Source: CAD feature listing. Evaluate the final solid. Frame: model axes, mm. A direction names the side the tool comes from. Round coordinates to 2 decimals unless told otherwise and drop trailing zeros. Loops run counter-clockwise (first coordinate to the right, second up) from the corner with the lowest first, then second, coordinate; pieces in that order, holes last. Notation, with made-up numbers: (84.5, -36) - (140.5, -36) arc R15 cw to (140.5, -14) - close; hole circle Ø5 at (81, 21.5). An arc over 180 degrees is marked (long way). One line per question, with ' | ' between items. Start each with the question number.
1. Pin query (flat end, axial travel): pin 1 (6.5 mm diameter, centred on x = 0, z = -62.5, fed in from +Y); pin 2 (1 mm diameter, centred on x = 4.5, y = -22, fed in from -Z); pin 3 (4 mm diameter, centred on x = -22.5, y = -22.5, fed in from -Z); pin 4 (3 mm diameter, centred on y = 1, z = -37.5, fed in from +X). Return the tip coordinate at first contact, or that it passes through.
2. Cut plane D-D (x = 22.5). Return loops of the section in (y, z), then the cut area to 3 significant figures.
3. Access query for faces 4 (the flat face through (-27.5, -9.6, 0.4)), 5 (the flat face through (-27.5, -29, -61)), 6 (the flat face through (-14, 27.5, -37)). Directions: +Z, -Z, +X, -X, +Y, -Y. A direction counts if a zero-diameter tool reaches every point of the face in a straight line with its end or side. Return the directions, or none.
4. Ray query, line 1 (Z direction, x = 0, y = -28); line 2 (Y direction, x = -21, z = -20.5); line 3 (Z direction, x = -13.5, y = 21.5). Return the intervals inside material, ascending.
5. Cut plane C-C (z = -12.5). Return loops of the section in (x, y), then the cut area to 3 significant figures.
6. Cut plane B-B (y = 0). Return loops of the section in (x, z), then the cut area to 3 significant figures.
7. Mould query, pull axis Z, two halves, no side actions, for faces 1 (the flat face through (-19, 6, 0)), 2 (the cylindrical face through (0, -28, -65)), 3 (the flat face through (-27.5, 0, -37)). Classes: pulls with the +Z half, pulls with the -Z half, needs draft (parallel to the pull), parting line crosses it, or undercut.
8. Cut plane A-A (x = -22.5). Return loops of the section in (y, z).
Autodesk Inventor part; units mm, degrees
ref_plane "YZ Plane" through (0, 0, 0) normal (1, 0, 0) x (0, 1, 0)
ref_plane "XZ Plane" through (0, 0, 0) normal (0, 1, 0) x (-1, 0, 0)
ref_plane "XY Plane" through (0, 0, 0) normal (0, 0, 1) x (1, 0, 0)
sketch "Sketch1" plane through (0, 0, 0) normal (0, 0, 1) x (1, 0, 0)
  line L0 (-27.5, 27.5) -> (27.5, 27.5)
  line L1 (27.5, 27.5) -> (27.5, -27.5)
  line L2 (27.5, -27.5) -> (-27.5, -27.5)
  line L3 (-27.5, -27.5) -> (-27.5, 27.5)
  circle A0 centre (-22.5, 22.5) radius 2.5
  circle A1 centre (22.5, 22.5) radius 2.5
  circle A2 centre (-22.5, -22.5) radius 2.5
  circle A3 centre (22.5, -22.5) radius 2.5
  circle A4 centre (0, 0) radius 19.25
  dimension "d1" = 55
  dimension "d2" = 55
  dimension "d3" = 27.5
  dimension "d4" = 27.5
  dimension "d5" = 38.5
  dimension "d6" = 5
  dimension "d7" = 5
  dimension "d8" = 5
  dimension "d9" = 5
  dimension "d10" = 5
  dimension "d11" = 5
  dimension "d12" = 5
  dimension "d13" = 5
  dimension "d14" = 5
  dimension "d15" = 5
  dimension "d16" = 5
  dimension "d17" = 5
extrude "Extrusion1" add sketch "Sketch1" along normal blind 2
sketch "Sketch2" plane through (27.5, -27.5, 0) normal (1, 0, 0) x (0, 0, -1)
  line L0 (0, 0) -> (-2, 0)
  line L1 (0, 0) -> (75, 0)
  line L2 (75, 0) -> (75, -2)
  line L3 (75, -2) -> (-2, -2)
  line L4 (-2, -2) -> (-2, 0)
  point P0 (0, 27.5)
  dimension "d20" = 75
  dimension "d21" = 2
  dimension "d22" = 77
extrude "Extrusion2" add sketch "Sketch2" against normal blind 55
sketch "Sketch3" plane through (-27.5, -27.5, 0) normal (-1, 0, 0) x (0, 0, 1)
  line L0 (-75, -2) -> (2, -2)
  line L1 (-36.5, -2) -> (-36.5, 55)
  line L2 (0, 0) -> (-75, 0)
  line L3 (-36.5, 55) -> (-46.5, 55)
  line L4 (-46.5, 55) -> (-46.5, -2)
  line L5 (-46.5, -2) -> (-26.5, -2)
  line L6 (-26.5, -2) -> (-26.5, 55)
  line L7 (-26.5, 55) -> (-36.5, 55)
  point P0 (0, 27.5)
  dimension "d25" = 57
  dimension "d26" = 10
  dimension "d27" = 57
  dimension "d28" = 20
  dimension "d29" = 57
extrude "Extrusion3" add sketch "Sketch3" along normal blind 2
sketch "Sketch4" plane through (-27.5, 27.5, -26.5) normal (0, 1, 0) x (1, 0, 0)
  line L0 (-2, 0) -> (-2, 20)
  line L1 (-2, 20) -> (27.5, 20)
  line L2 (27.5, 20) -> (27.5, 0)
  line L3 (0, 0) -> (-2, 0)
  line L4 (27.5, 0) -> (-2, 0)
  line L5 (-2, 0) -> (-2, 20)
  point P0 (27.5, -26.5)
  dimension "d32" = 29.5
  dimension "d33" = 20
extrude "Extrusion4" add sketch "Sketch4" along normal blind 2
sketch "Sketch5" plane through (27.5, -27.5, 0) normal (0, 1, 0) x (1, 0, 0)
  line L0 (0, 75) -> (0, 0)
  line L1 (0, 37.5) -> (-27.5, 37.5)
  line L2 (-27.5, 37.5) -> (-27.5, 62.5)
  line L3 (-27.5, 26.5) -> (-27.5, 46.5)
  line L4 (-27.5, 37.5) -> (-27.5, 12.5)
  circle A0 centre (-27.5, 62.5) radius 2.5
  circle A1 centre (-27.5, 12.5) radius 2.5
  point P0 (-27.5, 0)
  dimension "d36" = 27.5
  dimension "d37" = 25
  dimension "d38" = 25
  dimension "d39" = 5
  dimension "d40" = 5
extrude "Extrusion5" cut sketch "Sketch5" against normal blind 2
equation "\"BendRadius\" = Thickness"
equation "\"BendReliefWidth\" = Thickness"
equation "\"BendReliefDepth\" = 0.5 * Thickness"
equation "\"CornerReliefSize\" = 4 * Thickness"
equation "\"MinimumRemnant\" = 2 * Thickness"
equation "\"TransitionRadius\" = BendRadius"
equation "\"JacobiRadiusSize\" = Thickness"
equation "\"GapSize\" = Thickness"
properties part number "MotorClamp"
Answers follow:
1) pin 1: stops at y = -27.5 | pin 2: stops at z = 0 | pin 3: passes through | pin 4: stops at x = -27.5
2) outline: (-29.5, -75) - (-27.5, -75) - (-27.5, 0) - (-25, 0) - (-25, 2) - (-29.5, 2) - close; (-20, 0) - (20, 0) - (20, 2) - (-20, 2) - close; (25, 0) - (27.5, 0) - (27.5, 2) - (25, 2) - close | area: 244 mm2
3) face 4: +Z, -X, +Y, -Y | face 5: -Z, -X, +Y, -Y | face 6: -Z, +X
4) line 1: z = -75 to -65, -60 to -15, -10 to 2 | line 2: y = -29.5 to -27.5 | line 3: z = 0 to 2
5) outline: (-27.5, -29.5) - (-2.5, -29.5) - (-2.5, -27.5) - (-27.5, -27.5) - close; (2.5, -29.5) - (27.5, -29.5) - (27.5, -27.5) - (2.5, -27.5) - close | area: 100 mm2
6) outline: (-29.5, -46.5) - (-27.5, -46.5) - (-27.5, -26.5) - (-29.5, -26.5) - close; (-27.5, 0) - (-19.25, 0) - (-19.25, 2) - (-27.5, 2) - close; (19.25, 0) - (27.5, 0) - (27.5, 2) - (19.25, 2) - close | area: 73.0 mm2
7) face 1: pulls with the -Z half | face 2: undercut | face 3: needs draft
8) outline: (-29.5, -75) - (-27.5, -75) - (-27.5, 0) - (-25, 0) - (-25, 2) - (-29.5, 2) - close; (-20, 0) - (20, 0) - (20, 2) - (-20, 2) - close; (25, 0) - (27.5, 0) - (27.5, 2) - (25, 2) - close; (27.5, -46.5) - (29.5, -46.5) - (29.5, -26.5) - (27.5, -26.5) - close
